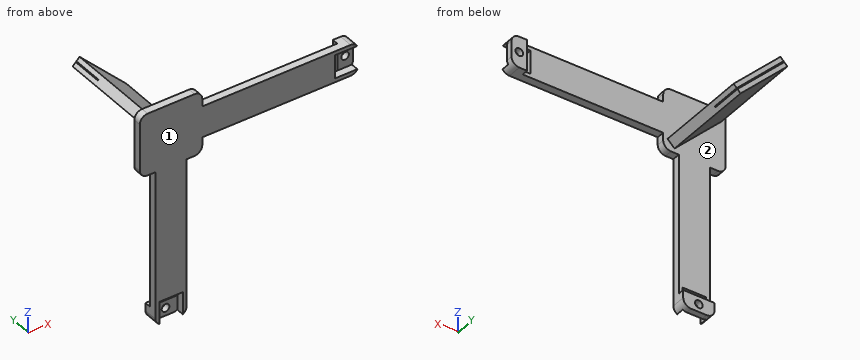
Autodesk Inventor part; units mm, degrees
ref_plane "Work Plane1" through (48.9401, 6.35, -48.9401) normal (-0.7071, 0, -0.7071) x (0, -1, 0)
ref_plane "YZ Plane" through (0, 0, 0) normal (1, 0, 0) x (0, 1, 0)
ref_plane "XZ Plane" through (0, 0, 0) normal (0, 1, 0) x (-1, 0, 0)
sketch "Sketch1" plane through (0, 0, 0) normal (0, 1, 0) x (-1, 0, 0)
  line L0 (-6.35, 0) -> (-44.45, 0)
  line L1 (0, -44.45) -> (0, -6.35)
  line L2 (-38.1, -50.8) -> (-38.1, -171.45)
  line L3 (-31.75, -177.8) -> (-19.05, -177.8)
  line L4 (-12.7, -171.45) -> (-12.7, -50.8)
  line L5 (-25.4, 0) -> (-25.4, -50.8) construction
  line L6 (-44.45, -50.8) -> (-25.4, -50.8)
  line L7 (-12.7, -50.8) -> (-6.35, -50.8)
  line L8 (0, 0) -> (-50.8, -50.8) construction
  line L9 (-50.8, -38.1) -> (-171.45, -38.1)
  line L10 (-177.8, -31.75) -> (-177.8, -19.05)
  line L11 (-171.45, -12.7) -> (-50.8, -12.7)
  line L12 (-50.8, -6.35) -> (-50.8, -12.7)
  line L13 (-50.8, -38.1) -> (-50.8, -44.45)
  arc A0 (-50.8, -44.45) -> (-44.45, -50.8) centre (-44.45, -44.45) ccw
  arc A1 (-6.35, -50.8) -> (0, -44.45) centre (-6.35, -44.45) ccw
  arc A2 (0, -6.35) -> (-6.35, 0) centre (-6.35, -6.35) ccw
  arc A3 (-44.45, 0) -> (-50.8, -6.35) centre (-44.45, -6.35) ccw
  arc A4 (-19.05, -177.8) -> (-12.7, -171.45) centre (-19.05, -171.45) ccw
  arc A5 (-38.1, -171.45) -> (-31.75, -177.8) centre (-31.75, -171.45) ccw
  arc A6 (-171.45, -12.7) -> (-177.8, -19.05) centre (-171.45, -19.05) ccw
  arc A7 (-177.8, -31.75) -> (-171.45, -38.1) centre (-171.45, -31.75) ccw
  point P0 (-50.8, 0)
  point P1 (0, -50.8)
  point P2 (-38.1, -177.8)
  point P3 (-12.7, -177.8)
  point P4 (-177.8, -38.1)
  point P5 (-177.8, -12.7)
  dimension "d0" = 50.8
  dimension "d1" = 50.8
  dimension "d2" = 25.4
  dimension "d3" = 127
  dimension "d4" = 6.35
  dimension "d5" = 6.35
  dimension "d6" = 6.35
extrude "Extrusion2" add sketch "Sketch1" along normal blind 6.35
sketch "Sketch2" plane through (0, 6.35, 0) normal (0, 1, 0) x (1, 0, 0)
  arc A0 (50.8, 44.45) -> (44.45, 50.8) centre (44.45, 44.45) ccw construction
  arc A1 (0, 6.35) -> (6.35, 0) centre (6.35, 6.35) ccw construction
  line L0 (44.45, 44.45) -> (6.35, 6.35) construction
  line L1 (6.6306, 6.0694) -> (44.7306, 44.1694)
  line L2 (6.6306, 6.0694) -> (9.1706, 3.5294)
  line L3 (9.1706, 3.5294) -> (47.2706, 41.6294)
  line L4 (44.7306, 44.1694) -> (47.2706, 41.6294)
  line L5 (6.0694, 6.6306) -> (44.1694, 44.7306)
  line L6 (6.0694, 6.6306) -> (3.5294, 9.1706)
  line L7 (3.5294, 9.1706) -> (41.6294, 47.2706)
  line L8 (44.1694, 44.7306) -> (41.6294, 47.2706)
  point P0 (0, 0)
  dimension "d14" = 38.1
  dimension "d15" = 0.3969
  dimension "d16" = 0.2806
  dimension "d17" = 90
  dimension "d18" = 2.54
extrude "Extrusion3" add sketch "Sketch2" along normal blind 76.2
sketch "Sketch3" plane through (0, 6.35, 0) normal (0, 1, 0) x (1, 0, 0)
  line L0 (6.0694, 6.6306) -> (44.1694, 44.7306)
  line L1 (47.2706, 41.6294) -> (44.7306, 44.1694)
  line L2 (44.1694, 44.7306) -> (44.7306, 44.1694)
  line L3 (44.7306, 44.1694) -> (6.6306, 6.0694)
  line L4 (44.7306, 44.1694) -> (6.6306, 6.0694)
  line L5 (6.0694, 6.6306) -> (3.5294, 9.1706)
  line L6 (6.6306, 6.0694) -> (6.0694, 6.6306)
  line L7 (6.0694, 6.6306) -> (44.1694, 44.7306)
  point P0 (0, 0)
extrude "Extrusion4" add sketch "Sketch3" along normal blind 50.8
sketch "Sketch4" plane through (0, 6.35, 0) normal (0, 1, 0) x (1, 0, 0)
  arc A0 (19.05, 177.8) -> (12.7, 171.45) centre (19.05, 171.45) ccw construction
  arc A1 (38.1, 171.45) -> (31.75, 177.8) centre (31.75, 171.45) ccw construction
  line L0 (19.05, 171.45) -> (31.75, 171.45) construction
  circle A2 centre (25.4, 171.45) radius 3.1386
  line L1 (12.7, 171.45) -> (12.7, 50.8)
  line L2 (12.7, 165.1) -> (38.1, 165.1)
  line L3 (38.1, 165.1) -> (38.1, 171.45)
  line L4 (12.7, 165.1) -> (12.7, 171.45)
  line L5 (31.75, 177.8) -> (19.05, 177.8)
  line L6 (19.05, 177.8) -> (31.75, 177.8)
  arc A3 (19.05, 177.8) -> (12.7, 171.45) centre (19.05, 171.45) ccw
  arc A4 (38.1, 171.45) -> (31.75, 177.8) centre (31.75, 171.45) ccw
  point P0 (0, 0)
  point P1 (14.5599, 175.9401)
  dimension "d23" = 6.2773
  dimension "d68" = 6.35
ref_plane "Work Plane1" through (48.9401, 6.35, -48.9401) normal (-0.7071, 0, -0.7071) x (0, -1, 0)
extrude "Extrusion6" add sketch "Sketch4" along normal blind 5.08
sketch "Sketch11" plane through (0, 0, 0) normal (0, -1, 0) x (1, 0, 0)
  line L0 (34.925, -177.8) -> (15.875, -177.8) construction
  line L1 (25.4, -177.8) -> (25.4, -169.6336) construction
  line L2 (34.925, -177.8) -> (15.875, -177.8)
  line L3 (15.875, -177.8) -> (15.875, -158.75)
  line L4 (15.875, -158.75) -> (34.925, -158.75)
  line L5 (34.925, -158.75) -> (34.925, -177.8)
  line L6 (31.75, -177.8) -> (19.05, -177.8)
  point P0 (0, 0)
  dimension "d71" = 19.05
  dimension "d74" = 19.05
extrude "Extrusion7" cut sketch "Sketch11" against normal blind 6.35
mirror "Mirror2" about plane through (48.9401, 6.35, -48.9401) normal (-0.7071, 0, -0.7071) of "Extrusion6", "Extrusion7"
equation "\"d37\" = 55deg"
equation "\"Sketch5_Pitch\" = 1.27"
equation "\"d56\" = 55deg"
equation "\"Sketch8_Pitch\" = 1.27"
properties part number "beamsplitter main"
Source: CAD feature listing. Evaluate the final solid. Frame: model axes, mm. Face numbers are marked on the shaded views. Round coordinates to 2 decimals unless told otherwise and drop trailing zeros. Loops run counter-clockwise (first coordinate to the right, second up) from the corner with the lowest first, then second, coordinate; pieces in that order, holes last. Notation, with made-up numbers: M -37,72.25 L -1,72.25 A8 cw -1,85.25 Z; hole C 18,-34.75 d2. An arc over 180 degrees is marked long. Return JSON: item names as keys, results as strings. Group by question number.
1. Material intervals for line 1 along X through (y, z) = (8, -25); line 2 along X through (y, z) = (7.45, -171.45); line 3 along Z through (x, y) = (171.45, 9.15), sorted ascending. Write a range as from..to.
2. Section query C-C on y = 51.5. Output: boundary loops of the cut face in (x, z).
3. Section query D-D on x = 100. Output: boundary loops of the cut face in (y, z), and give its area (3 significant figures).
4. Section query B-B on x = 25.4. Output: boundary loops of the cut face in (y, z), and give its area (3 significant figures).
5. Pin query (flat end, axial travel): pin 1 (3.5 mm diameter, centred on x = 97.5, y = 3.5, fed in from +Z); pin 2 (12 mm diameter, centred on y = 38, z = -34.5, fed in from +X); pin 3 (1.5 mm diameter, centred on x = 25.5, y = 9.5, fed in from +Z). Return the tip coordinate at first contact, or that it passes through.
6. Mould query, pull axis Z, two halves, no side actions, for the marked faces 1 and 2. Classes: released by +Z, released by -Z, zero draft, split by the parting line, or undercut.
7. Section query A-A on z = -25.4. Output: boundary loops of the cut face in (x, y), and give its area (3 significant figures).
Checks:
{
 "1": {"line 1": "x = 19.36..30.64, 165.1..168.34, 174.56..177.8", "line 2": "x = 12.7..22.26, 28.54..38.1", "line 3": "z = -38.1..-28.54, -22.26..-12.7"},
 "2": {"outline": "M 3.53,-9.17 L 41.63,-47.27 L 47.27,-41.63 L 9.17,-3.53 Z"},
 "3": {"outline": "M 0,-38.1 L 6.35,-38.1 L 6.35,-12.7 L 0,-12.7 Z", "area": "161 mm²"},
 "4": {"outline": "M 0,-158.75 L 6.35,-158.75 L 6.35,-31.04 L 82.55,-31.04 L 82.55,-25.96 L 57.15,-25.96 L 57.15,-24.84 L 82.55,-24.84 L 82.55,-19.76 L 6.35,-19.76 L 6.35,0 L 0,0 Z; M 6.35,-177.8 L 11.43,-177.8 L 11.43,-174.59 L 6.35,-174.59 Z; M 6.35,-168.31 L 11.43,-168.31 L 11.43,-165.1 L 6.35,-165.1 Z", "area": "1,870 mm²"},
 "5": {"pin 1": "stops at z = -12.7", "pin 2": "stops at x = 46.14", "pin 3": "stops at z = -19.11"},
 "6": {"face 1": "zero draft", "face 2": "undercut"},
 "7": {"outline": "M 0,0 L 158.75,0 L 158.75,6.35 L 31.04,6.35 L 31.04,82.55 L 25.96,82.55 L 25.96,57.15 L 24.84,57.15 L 24.84,82.55 L 19.76,82.55 L 19.76,6.35 L 0,6.35 Z; M 165.1,6.35 L 168.31,6.35 L 168.31,11.43 L 165.1,11.43 Z; M 174.59,6.35 L 177.8,6.35 L 177.8,11.43 L 174.59,11.43 Z", "area": "1,870 mm²"}
}
